Can you work these out from the drawing? Everything is in mm from the part's minimum corner. A direction names the side the tool comes from. Coordinates: 2 decimals unless noted, no trailing zeros. Order: outer loops, then holes, each group sorted by start corner. A loop starts at its lowest first (then second) coordinate and runs counter-clockwise, first axis right, second up. Notation, with made-up numbers: (30.25, 73.25) - (63.25, 73.25) arc R15 ccw to (63.25, 101.25) - close; hole circle Ø7 at (53, 40). An arc over 180 degrees is marked (long way). One line per item, written item: value.
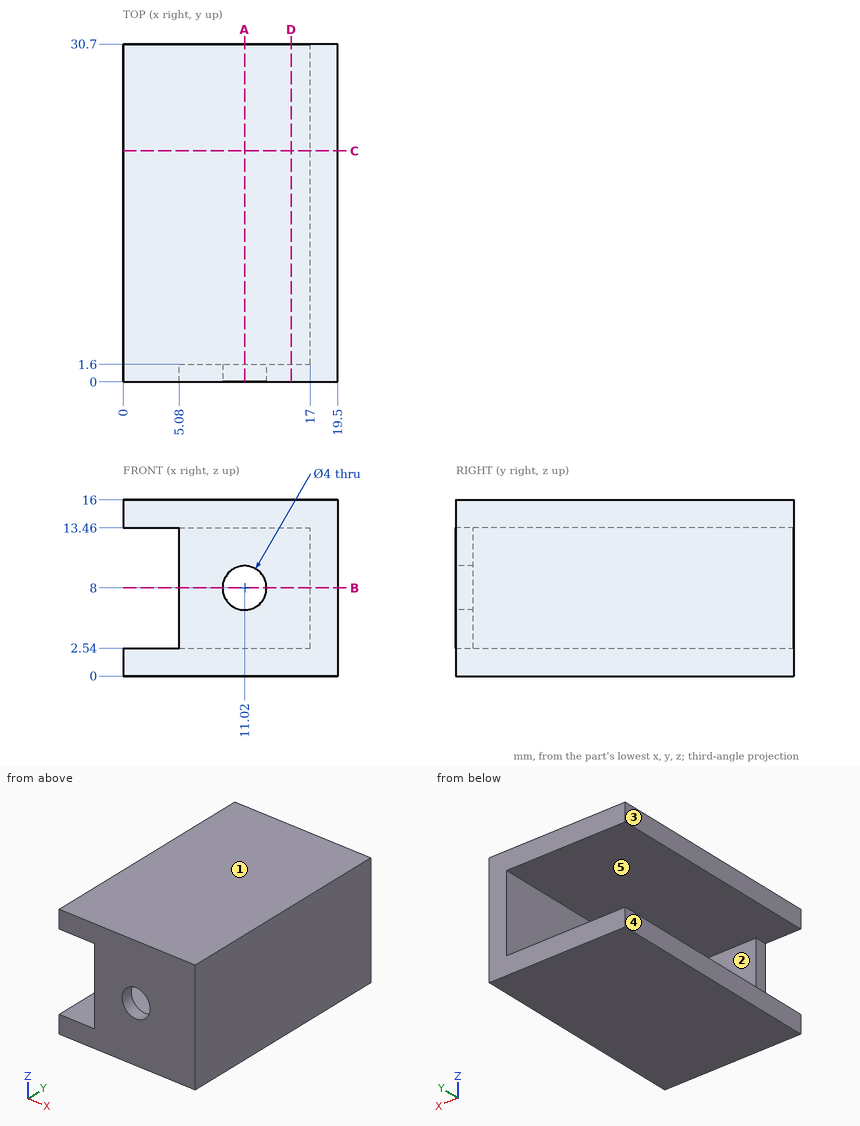
Item 1: Thinking about a two-plate mould opening in Z: for the marked faces 1, 2 and 3, which applies, pulls with the +Z half, pulls with the -Z half, needs draft (parallel to the pull), parting line crosses it, or undercut?
Conclusion:
face 1: pulls with the +Z half
face 2: undercut
face 3: needs draft
Item 2: I want a section at B-B on z = 8. Please give me the cut outline in (x, y), then the cut area to 3 significant figures.
Conclusion:
outline: (5.08, 0) - (9.02, 0) - (9.02, 1.6) - (5.08, 1.6) - close; (13.02, 0) - (19.5, 0) - (19.5, 30.7) - (17, 30.7) - (17, 1.6) - (13.02, 1.6) - close
area: 89.4 mm²
Item 3: I want a section at C-C on y = 21. Please give me the cut outline in (x, z), then the cut area to 3 significant figures.
Conclusion:
outline: (0, 0) - (19.5, 0) - (19.5, 16) - (0, 16) - (0, 13.46) - (17, 13.46) - (17, 2.54) - (0, 2.54) - close
area: 126 mm²
Item 4: For the marked faces 4 and 5, which set-ups out of +Z, -Z, +X, -X, +Y, -Y let a thin tool reach every point of the face, with its end or its side?
Conclusion:
face 4: +Z, -Z, -X, +Y, -Y
face 5: -X, +Y
Item 5: I want a section at A-A on x = 11.02. Please give me the cut outline in (y, z), then the cut area to 3 significant figures.
Conclusion:
outline: (0, 0) - (30.7, 0) - (30.7, 2.54) - (1.6, 2.54) - (1.6, 6) - (0, 6) - close; (0, 10) - (1.6, 10) - (1.6, 13.46) - (30.7, 13.46) - (30.7, 16) - (0, 16) - close
area: 167 mm²
Item 6: I want a section at D-D on x = 15.25. Please give me the cut outline in (y, z), then the cut area to 3 significant figures.
Conclusion:
outline: (0, 0) - (30.7, 0) - (30.7, 2.54) - (1.6, 2.54) - (1.6, 13.46) - (30.7, 13.46) - (30.7, 16) - (0, 16) - close
area: 173 mm²
Item 7: If I drill on probe 1 along Z at (x, y) = (3.75, 20.5); probe 2 along Z at (x, y) = (11.02, 1.2); probe 3 along Y at (x, z) = (16.5, 7), over which ranges is the centre line in solid material (lowest first)?
Conclusion:
probe 1: 0 to 2.54, 13.46 to 16
probe 2: 0 to 6, 10 to 16
probe 3: 0 to 1.6
Item 8: I'm going to push flat-ended pins straight in: pin 1 Ø3.5 at (y, z) = (14, 8.5) entering from -X; pin 2 Ø2.5 at (x, z) = (11.02, 8) entering from -Y; pin 3 Ø0.5 at (y, z) = (1, 7) entering from -X. Where does each tip first touch, or does it pass through?
Conclusion:
pin 1: x = 17
pin 2: through
pin 3: x = 5.08
